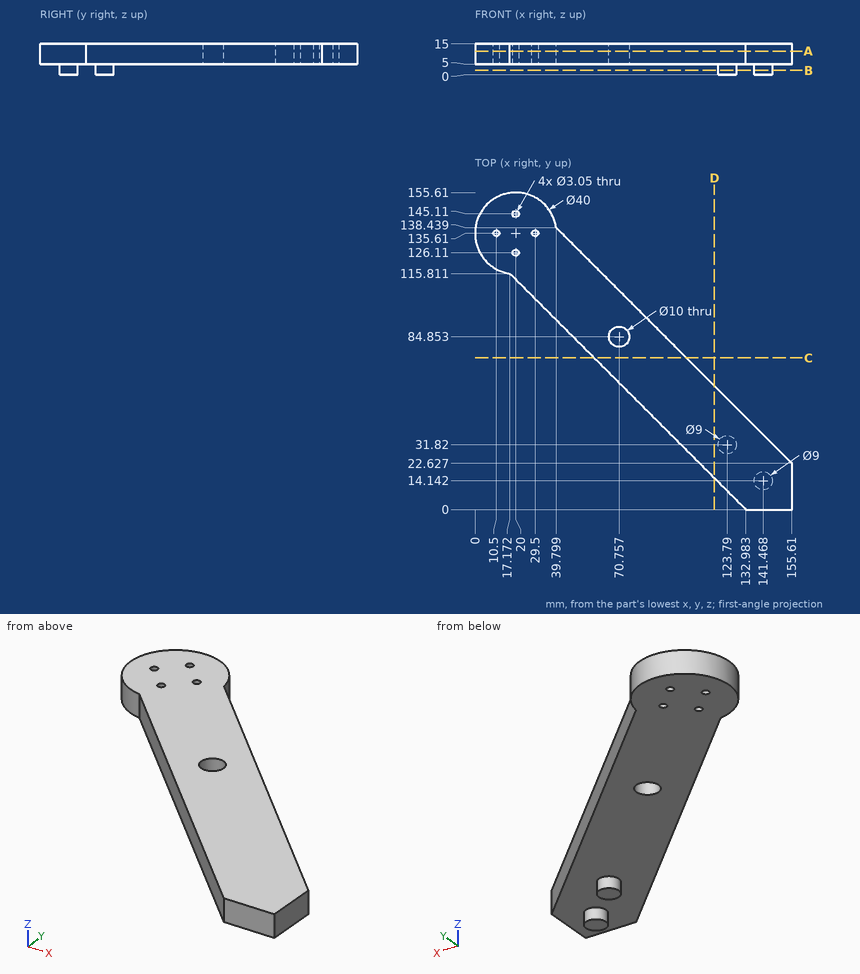
Study the drawing (mm; zero at the part's minimum x, y, z) and answer. Coordinates: 2 decimals unless noted, no trailing zeros. Write each loop counter-clockwise with the first axis right and the second up, starting at its lowest first coordinate (ties: lowest second). Pieces come first, ordered by that corner, then holes.
Q1. Section B-B, the plane z = 2 is taken. Write down the section's boundary in (x, y), then the cut area to 3 significant figures.
Returned:
outline: circle Ø9 at (123.79, 31.82); circle Ø9 at (141.47, 14.14)
area: 127 mm2
Q2. Section C-C, the plane y = 74.5 is taken. Write down the section's boundary in (x, z).
Returned:
outline: (58.48, 5) - (103.74, 5) - (103.74, 15) - (58.48, 15) - close
Q3. Section D-D, the plane x = 117.5 is taken. Write down the section's boundary in (y, z).
Returned:
outline: (15.48, 5) - (60.74, 5) - (60.74, 15) - (15.48, 15) - close
Q4. Section A-A, the plane z = 11.5 is taken. Give the number of separate pieces and of enclosed holes in the cut face, then the cut area to 3 significant figures.
Returned:
separate pieces: 1
enclosed holes: 5
area: 6,470 mm2
Q5. Find the intervals of material crossed by line 1 along Y through (x, z) = (20, 10) (1 decimal); line 2 along Z through (x, y) = (47, 101.5); line 3 along Y through (x, z) = (29.5, 8.75) (1 decimal), in increasing order.
Returned:
line 1: y = 113 to 124.6, 127.6 to 143.6, 146.6 to 155.6
line 2: z = 5 to 15
line 3: y = 103.5 to 134.1, 137.1 to 153.2
Q6. Given P1, Ø3, axis at x = 138, z = 12.5, coming from the +Y side; P2, Ø5, axis at x = 53.5, z = 7.5, coming from the -Y side; P3, Ø6, axis at x = 75, y = 101, coming from the -Z side, each flat-ended and moving along its own axis, determine where each tip first touches the part or whether it passes through.
Returned:
P1: stops at y = 41.74
P2: stops at y = 76.98
P3: stops at z = 5
